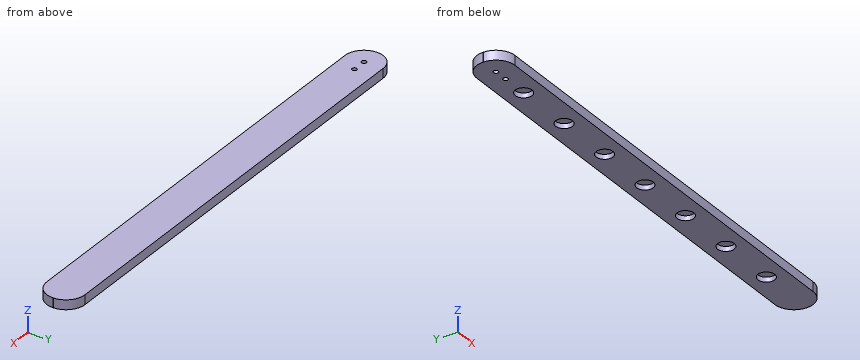
```python
from build123d import *

# Parameters (mm, degrees)
BOSS_EXTRUDE1_DEPTH = 19.05
SKETCH3_R           = 16.66875
CUT_EXTRUDE1_DEPTH  = 9.525
SKETCH5_R           = 4.9609375
SKETCH5_R_2         = 4.7625
CUT_EXTRUDE10_DEPTH = 19.05


with BuildPart() as part:
    # Sketch2 → Boss-Extrude1 (new body)
    with BuildSketch(Plane.XY):
        with BuildLine():
            Line((37.846, 0), (927.354, 0))
            ThreePointArc((927.354, 0), (954.115163241, -11.084836759), (965.2, -37.846))
            Line((965.2, -37.846), (965.2, -38.354))
            ThreePointArc((965.2, -38.354), (954.115163241, -65.115163241), (927.354, -76.2))
            Line((927.354, -76.2), (37.846, -76.2))
            ThreePointArc((37.846, -76.2), (11.084836759, -65.115163241), (0, -38.354))
            Line((0, -38.354), (0, -37.846))
            ThreePointArc((0, -37.846), (11.084836759, -11.084836759), (37.846, 0))
        make_face()
    extrude(amount=BOSS_EXTRUDE1_DEPTH)

    # Sketch3 → Cut-Extrude1 (cut)
    with BuildSketch(Plane.XY):
        with Locations((120.65, -38.1)):
            Circle(SKETCH3_R)
        with Locations((241.3, -38.1)):
            Circle(SKETCH3_R)
        with Locations((361.95, -38.1)):
            Circle(SKETCH3_R)
        with Locations((844.55, -38.1)):
            Circle(SKETCH3_R)
        with Locations((723.9, -38.1)):
            Circle(SKETCH3_R)
        with Locations((603.25, -38.1)):
            Circle(SKETCH3_R)
        with Locations((482.6, -38.1)):
            Circle(SKETCH3_R)
    extrude(amount=CUT_EXTRUDE1_DEPTH, mode=Mode.SUBTRACT)

    # Sketch5 → Cut-Extrude10 (cut)
    with BuildSketch(Plane.XY):
        with Locations((38.1, -38.1)):
            Circle(SKETCH5_R)
        with Locations((66.675, -38.1)):
            Circle(SKETCH5_R_2)
    extrude(amount=CUT_EXTRUDE10_DEPTH, mode=Mode.SUBTRACT)


solid = part.part
```
For this review, take the finished solid that the model builds, in its own axes (mm). Round coordinates to 2 decimals unless told otherwise and drop trailing zeros. Write each loop counter-clockwise with the first axis right and the second up, starting at its lowest first coordinate (ties: lowest second). Pieces come first, ordered by that corner, then holes. Notation, with made-up numbers: (20.5, 75) -> (28.5, 75) arc R19 cw to (28.5, 85) -> close; hole circle Ø7 at (43.25, 18). An arc over 180 degrees is marked (long way). One line per question, with ' | ' between items. Start each with the question number.
(1) Insertion check: P1, Ø2, axis at y = -64.5, z = 15, coming from the +X side; P2, Ø5, axis at y = -60, z = 4.5, coming from the +X side; P3, Ø1.5, axis at y = -35.5, z = 14.5, coming from the +X side. Each pin has a flat end and moves straight along its axis. Give the tip position at first contact, or say it passes through.
(2) Add section B-B, the plane x = 482.6. Write out the cut boundary in (y, z) (3 decimals), plus the area to 3 significant figures.
(3) For line 1 along Y through (x, z) = (361.95, 2.5); line 2 along Y through (x, z) = (38.1, 13.5); line 3 along Z through (x, y) = (853.5, -28) (3 decimals), list the stretches that pass through material, from the lowest coordinate up. Write a range as from..to.
(4) Add section C-C, the plane y = -10. Write out the cut boundary in (x, z).
(5) Add section A-A, the plane z = 12.5. Write out the cut boundary in (x, y) (1 decimal), plus the area to 3 significant figures.
Answer list:
1) P1: x = 955.64 | P2: x = 960 | P3: x = 965.17
2) outline: (-76.2, 0) -> (-54.769, 0) -> (-54.769, 9.525) -> (-21.431, 9.525) -> (-21.431, 0) -> (0, 0) -> (0, 19.05) -> (-76.2, 19.05) -> close | area: 1,130 mm²
3) line 1: -76.2..-54.77, -21.43..0 | line 2: -76.2..-43.06, -33.14..0 | line 3: 9.525..19.05
4) outline: (12.22, 0) -> (952.98, 0) -> (952.98, 19.05) -> (12.22, 19.05) -> close
5) outline: (0, -38.4) arc R37.8 ccw to (37.8, -76.2) -> (927.4, -76.2) arc R37.8 ccw to (965.2, -38.4) -> (965.2, -37.8) arc R37.8 ccw to (927.4, 0) -> (37.8, 0) arc R37.8 ccw to (0, -37.8) -> close; hole circle Ø9.9 at (38.1, -38.1); hole circle Ø9.5 at (66.7, -38.1) | area: 72,200 mm²
